Design review of the part built by this model. Coordinates are the model's own, in mm. Face numbers are marked on the shaded views. Round coordinates to 2 decimals unless told otherwise and drop trailing zeros. Loops run counter-clockwise (first coordinate to the right, second up) from the corner with the lowest first, then second, coordinate; pieces in that order, holes last. Notation, with made-up numbers: (80.25, 43.5) - (130.25, 43.5) arc R36 cw to (130.25, 79.5) - close; hole circle Ø9 at (-29.5, 73.25). An arc over 180 degrees is marked (long way). One line per question, with ' | ' between items. Start each with the question number.
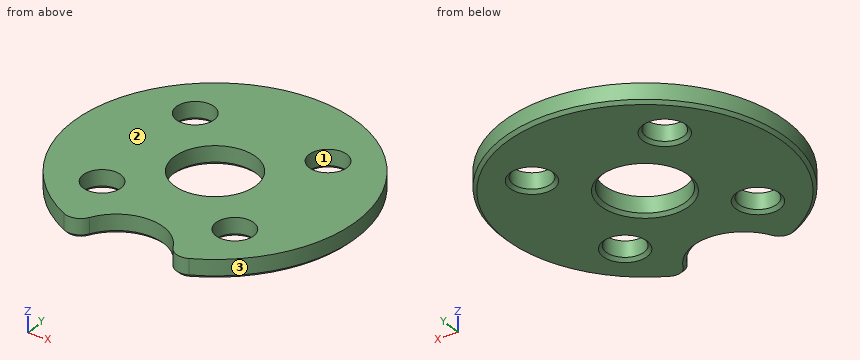
from build123d import *

# Parameters (mm, degrees)
F0_R     = 9
F0_R_2   = 1.2
F0_R_3   = 2.6
F2_R     = 3
F4_DEPTH = 1.201
F5_R     = 1
F6_SIZE  = 0.2


with BuildPart() as f3:
    # F3: sweep along a path in F1
    with BuildLine(Plane.XZ) as f3_path:
        Line((0, 0), (0, 1.2))
    # F0 (on Top) → F3 (sweep)
    with BuildSketch(Plane.XY):
        Circle(F0_R)
        with Locations((-4.2426406871, -4.2426406871)):
            Circle(F0_R_2, mode=Mode.SUBTRACT)
        with Locations((4.2426406871, -4.2426406871)):
            Circle(F0_R_2, mode=Mode.SUBTRACT)
        with Locations((-4.2426406871, 4.2426406871)):
            Circle(F0_R_2, mode=Mode.SUBTRACT)
        Circle(F0_R_3, mode=Mode.SUBTRACT)
        with Locations((4.2426406871, 4.2426406871)):
            Circle(F0_R_2, mode=Mode.SUBTRACT)
    sweep(path=f3_path.line)

    # F2 (on Top) → F4 (cut, through all)
    with BuildSketch(Plane.XY):
        with Locations((0, -9)):
            Circle(F2_R)
    extrude(amount=F4_DEPTH, mode=Mode.SUBTRACT)

    # F5
    f5_edges = [f3.edges().sort_by_distance(p)[0] for p in [
        (-2.95804, -8.5, 0.6),
        (2.95804, -8.5, 0.6),
    ]]
    fillet(f5_edges, radius=F5_R)

    # F6
    f6_edges = [f3.edges().sort_by_distance(p)[0] for p in [
        (0, 9, 0),
        (3.243317, -8.116813, 0),
        (-3.243317, -8.116813, 0),
        (0, -6, 0),
        (-5.442641, -4.242641, 0),
        (3.042641, -4.242641, 0),
        (-2.6, 0, 0),
        (-5.442641, 4.242641, 0),
        (3.042641, 4.242641, 0),
    ]]
    chamfer(f6_edges, length=F6_SIZE)


solid = f3.part
1. The part is to be moulded in two halves that separate along X. For the marked faces 1, 2 and 3, say which applies: pulls with the +X half, pulls with the -X half, needs draft (parallel to the pull), parting line crosses it, or undercut.
2. Take a section at C-C, the plane x = -3.25. Count the separate pieces of the cut face and the enclosed holes in it, then the cut area to 3 significant figures.
3. To check wall thickness, follow line 1 along Y through (x, z) = (0, 0.95); line 2 along Y through (x, z) = (-5.25, 0.4); line 3 along X through (y, z) = (-3.25, 0.5). State the ranges of each line that lie inside material, in increasing order.
4. Take a section at A-A, the plane x = 0. Give the boundary of the cut face in (y, z).
5. Take a section at B-B, the plane y = 0. Give the boundary of the cut face in (x, z).
Answer list:
1) face 1: undercut | face 2: needs draft | face 3: parting line crosses it
2) separate pieces: 3 | enclosed holes: 0 | area: 16.4 mm²
3) line 1: y = -6 to -2.6, 2.6 to 9 | line 2: y = -7.31 to -4.89, -3.59 to 3.59, 4.89 to 7.31 | line 3: x = -8.39 to -4.92, -3.57 to 3.57, 4.92 to 8.39
4) outline: (-6, 0.2) - (-5.8, 0) - (-2.8, 0) - (-2.6, 0.2) - (-2.6, 1.2) - (-6, 1.2) - close; (2.6, 0.2) - (2.8, 0) - (8.8, 0) - (9, 0.2) - (9, 1.2) - (2.6, 1.2) - close
5) outline: (-9, 0.2) - (-8.8, 0) - (-2.8, 0) - (-2.6, 0.2) - (-2.6, 1.2) - (-9, 1.2) - close; (2.6, 0.2) - (2.8, 0) - (8.8, 0) - (9, 0.2) - (9, 1.2) - (2.6, 1.2) - close
